Answer from the drawing. Dimensions are ordinates in mm from the lowest x, y and z of the part. A direction names the side the tool comes from. Coordinates: 2 decimals unless noted, no trailing zeros. Write each loop counter-clockwise with the first axis right and the second up, starting at its lowest first coordinate (ties: lowest second). Pieces come first, ordered by that corner, then holes.
1) The part is cut by section B-B (y = 131). Determine the outline of the cut face in (x, z).
2) Each of these flat-tipped pins is pushed along its axis until it touches: pin 1 Ø6 at (x, z) = (40.5, 124.5) entering from -Y; pin 2 Ø10 at (x, y) = (254, 206.5) entering from +Z; pin 3 Ø2 at (x, z) = (240.5, 126.5) entering from -Y (1 decimal). Where does it stop, or does it pass through?
3) Which of the six approach directions +Z, -Z, +X, -X, +Y, -Y give full straight-line access (tool end or side, diameter ignored) to the marked faces 1 and 2?
4) The part is cut by section C-C (z = 233). Determine the outline of the cut face in (x, y), then the cut area to 3 significant figures.
5) Find the intervals of material crossed by line 1 (Y direction, x = 234, z = 204); line 2 (Z direction, x = 109, y = 910); line 3 (Z direction, x = 205, y = 395.5), in increasing order.
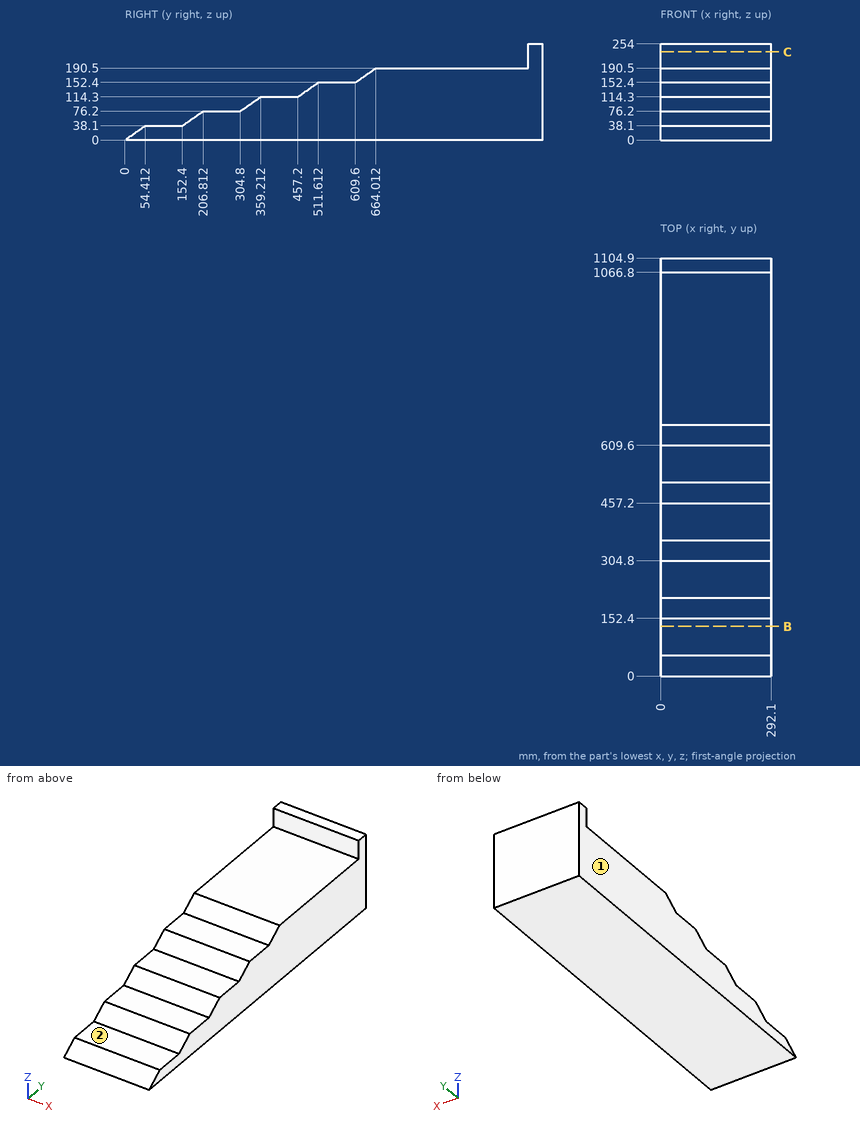
Reported:
1. outline: (0, 0) - (292.1, 0) - (292.1, 38.1) - (0, 38.1) - close
2. pin 1: stops at y = 467.48
2. pin 2: stops at z = 76.2
2. pin 3: stops at y = 473.2
3. face 1: +Z, -Z, -X, +Y, -Y
3. face 2: +Z, +X, -X, -Y
4. outline: (0, 1066.8) - (292.1, 1066.8) - (292.1, 1104.9) - (0, 1104.9) - close
4. area: 11,100 mm2
5. line 1: y = 1066.8 to 1104.9
5. line 2: z = 0 to 190.5
5. line 3: z = 0 to 114.3
